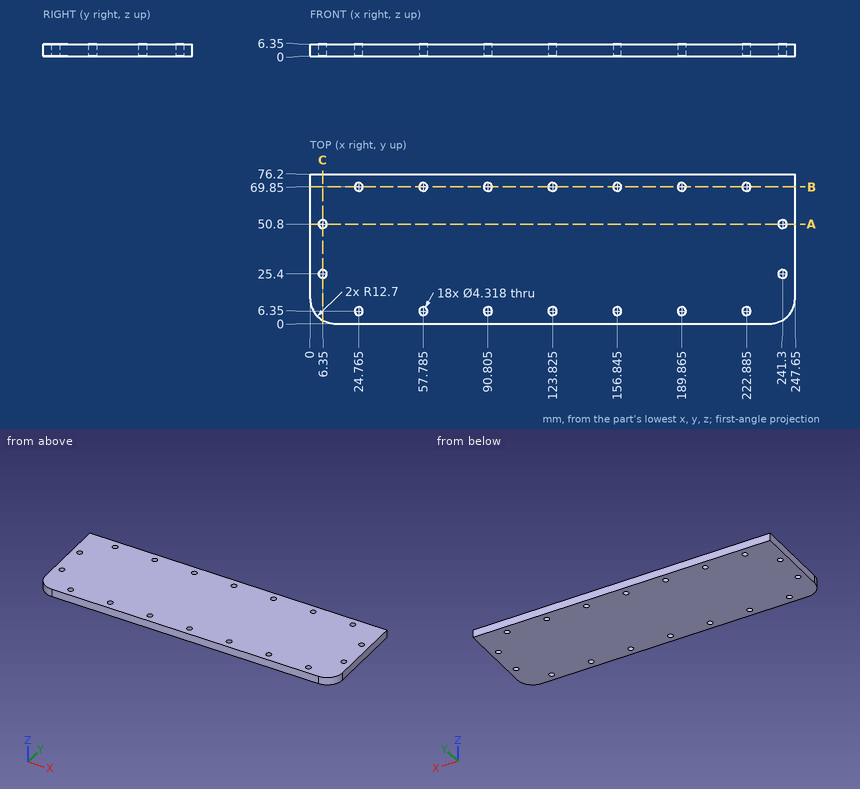
Here's the drawing with two shaded views (mm, measured from the low corner). I have some questions. Round coordinates to 2 decimals unless told otherwise and drop trailing zeros. Loops run counter-clockwise (first coordinate to the right, second up) from the corner with the lowest first, then second, coordinate; pieces in that order, holes last. Notation, with made-up numbers: (-35.75, -30) - (-19.75, -30) arc R21 cw to (-19.75, 8) - close; hole circle Ø3 at (60.25, -38). An arc over 180 degrees is marked (long way). Write item = value, one per line.
1) Imagine slicing it at A-A (y = 50.8). Please give me the cut outline in (x, z), and give its area (3 significant figures).
Computed:
outline = (0, 0) - (4.19, 0) - (4.19, 6.35) - (0, 6.35) - close; (8.51, 0) - (239.14, 0) - (239.14, 6.35) - (8.51, 6.35) - close; (243.46, 0) - (247.65, 0) - (247.65, 6.35) - (243.46, 6.35) - close
area = 1,520 mm2
2) I need wall thicknesses on line 1 along Y through (x, z) = (6.35, 5); line 2 along Y through (x, z) = (190, 5); line 3 along X through (y, z) = (12, 5.25). Which ranges of each line are inside material? Lowest first, please. Write a range as from..to.
Computed:
line_1 = 1.7..23.24, 27.56..48.64, 52.96..76.2
line_2 = 0..4.2, 8.5..67.7, 72..76.2
line_3 = 0.02..247.63
3) Imagine slicing it at C-C (x = 6.35). Please give me the cut outline in (y, z).
Computed:
outline = (1.7, 0) - (23.24, 0) - (23.24, 6.35) - (1.7, 6.35) - close; (27.56, 0) - (48.64, 0) - (48.64, 6.35) - (27.56, 6.35) - close; (52.96, 0) - (76.2, 0) - (76.2, 6.35) - (52.96, 6.35) - close
4) Imagine slicing it at B-B (y = 69.85). Give the number of separate pieces and of enclosed holes in the cut face, and give its area (3 significant figures).
Computed:
separate_pieces = 8
enclosed_holes = 0
area = 1,380 mm2
